Part model, mm, in its own coordinate system. A direction names the side the tool comes from. Give positions to 0.01 mm unless a question says otherwise; leave off trailing zeros. Use a Markdown table: item, result.
Autodesk Inventor part; units mm, degrees
ref_plane "Work Plane1" through (6.245, 5, -17) normal (0, 0, -1) x (-1, 0, 0)
ref_plane "YZ Plane" through (0, 0, 0) normal (1, 0, 0) x (0, 1, 0)
ref_plane "XY Plane" through (0, 0, 0) normal (0, 0, 1) x (1, 0, 0)
sketch "Sketch1" plane through (0, 0, 0) normal (0, 0, 1) x (1, 0, 0)
  point P0 (0, 0)
sketch "Sketch2" plane through (0, 0, 0) normal (1, 0, 0) x (0, 1, 0)
  line L0 (-13.0429, 0) -> (13.0429, 0)
  line L1 (13.0429, 0) -> (13.0429, 3.3095)
  line L2 (13.0429, 3.3095) -> (-13.0429, 3.3095)
  line L3 (-13.0429, 3.3095) -> (-13.0429, 0)
  line L4 (0, 0) -> (0, -15)
  line L5 (0, -15) -> (-8, -15)
  line L6 (-14.2875, 0) -> (14.2875, 0)
  line L7 (14.2875, 0) -> (14.2875, 6.8547)
  line L8 (14.2875, 6.8547) -> (-14.2875, 6.8547)
  line L9 (-14.2875, 6.8547) -> (-14.2875, 0)
  spline S0 degree 4 poles (-14.2875, 0) (-14.2875, -4.9566) (-13.3423, -10.7623) (-11.8115, -15) (-8, -15) knots 0 0 0 0 0 1 1 1 1 1
  point P0 (-12.3627, -11.4481)
  dimension "d1" = 26.0858
  dimension "d2" = 8
  dimension "d3" = 15
  dimension "d4" = 28.575
revolve "Revolution1" add sketch "Sketch2" angle 360 about axis through (0, 0, 0) along (0, 0, -1) contours L0 L4 L5 S0 L6
sketch "Sketch3" plane through (0, 0, 0) normal (0, 0, 1) x (1, 0, 0)
  circle A0 centre (0, 0) radius 14.2875
  circle A1 centre (0, 0) radius 13.0429
  circle A2 centre (0, 0) radius 11
  point P0 (0, -14.2875)
  dimension "d6" = 26.0858
  dimension "d7" = 22
extrude "Extrusion1" add sketch "Sketch3" along normal blind 5 contours A1
hole "Hole1" at (0, 0, 0) direction (0, 0, -1) diameter 3 end through all
sketch "Sketch6" plane through (0, 0, 0) normal (0, 0, 1) x (1, 0, 0)
  circle A0 centre (0, 0) radius 12
  point P0 (4.074, -8.737)
  point P1 (4.82, 8.349)
  point P2 (-9.494, -1.674)
  dimension "d22" = -8.737
  dimension "d23" = 8.349
  dimension "d24" = 1.674
  dimension "d25" = 4.074
  dimension "d26" = 4.82
hole "Hole2" at (-9.494, -1.674, 0) at (4.82, 8.349, 0) at (4.074, -8.737, 0) direction (0, 0, -1) diameter 1.7 end through all
sketch "Sketch8" plane through (0, 0, 0) normal (0, 1, 0) x (-1, 0, 0)
  point P0 (0, 0)
sketch "Sketch9" plane through (0, 0, -15) normal (0, 0, -1) x (-1, 0, 0)
  circle A0 centre (0, 0) radius 1.5
  line L0 (-10.3562, 5) -> (-3, 5)
  line L1 (-3, 5) -> (-3, -5)
  line L2 (-3, -5) -> (-10.3562, -5)
  line L3 (20.0025, 0) -> (-20.0025, 0)
  line L4 (0, -20.0025) -> (0, 20.0025)
  circle A1 centre (-4.82, 8.349) radius 0.85
  circle A2 centre (-4.074, -8.737) radius 0.85
  circle A3 centre (0, 0) radius 8
  arc A4 (-10.3562, 5) -> (-10.3562, -5) centre (0, 0) ccw
  point P0 (0, -8)
  point P1 (-10.7619, 0)
  dimension "d34" = 3
  dimension "d35" = 8.349
  dimension "d36" = 8.737
  dimension "d37" = 10
extrude "Extrusion2" cut sketch "Sketch9" against normal through all contours L3 A3 L0 L1 | L1 L2 A3 L3 | A3 L3 A4 L0 | L2 A4 L3 A3
sketch "Sketch10" plane through (6.245, 5, -15) normal (0, 0, -1) x (-1, 0, 0)
  arc A0 (2.1327, 3.8197) -> (2.1327, 3.8197) centre (2.1327, 3.8197) ccw
  arc A1 (3.0175, -13.6604) -> (3.0175, -13.6604) centre (3.0175, -13.6604) ccw
  arc A2 (16.4746, -6.2481) -> (16.4746, -6.2481) centre (16.4746, -6.2481) ccw
  circle A3 centre (1.425, 3.349) radius 0.85
  circle A4 centre (2.171, -13.737) radius 2.5
  circle A5 centre (2.171, -13.737) radius 0.85
  circle A6 centre (15.739, -6.674) radius 2.5
  circle A7 centre (15.739, -6.674) radius 0.85
  circle A8 centre (1.425, 3.349) radius 2.5
  dimension "d43" = 5
  dimension "d44" = 5
  dimension "d59" = 5
ref_plane "Work Plane1" through (6.245, 5, -17) normal (0, 0, -1) x (-1, 0, 0)
sketch "Sketch11" plane through (6.245, 5, -17) normal (0, 0, -1) x (-1, 0, 0)
  arc A0 (2.1327, 3.8197) -> (2.1327, 3.8197) centre (2.1327, 3.8197) ccw
  arc A1 (16.4746, -6.2481) -> (16.4746, -6.2481) centre (16.4746, -6.2481) ccw
  arc A2 (3.0175, -13.6604) -> (3.0175, -13.6604) centre (3.0175, -13.6604) ccw
  circle A3 centre (1.425, 3.349) radius 2.5
  circle A4 centre (1.425, 3.349) radius 0.85
  circle A5 centre (2.171, -13.737) radius 2.5
  circle A6 centre (15.739, -6.674) radius 2.5
  circle A7 centre (15.739, -6.674) radius 0.85
  circle A8 centre (2.171, -13.737) radius 0.85
  point P0 (6.245, -5)
  dimension "d61" = 5
  dimension "d62" = 5
  dimension "d63" = 5
hole "Hole5" at (4.82, 8.349, -17) at (-9.494, -1.674, -17) at (4.074, -8.737, -17) direction (0, 0, 1) diameter 5 depth 10
sketch "Sketch12" plane through (-9.494, -1.674, -7) normal (0, 0, -1) x (-1, 0, 0)
  circle A0 centre (0, 0) radius 0.85
  circle A1 centre (-14.314, 10.023) radius 0.85
  circle A2 centre (-13.568, -7.063) radius 0.85
  line L0 (-12.264, 8.8394) -> (-14.3141, 7.6559)
  line L1 (-14.3141, 7.6559) -> (-16.364, 8.8395)
  line L2 (-16.364, 8.8395) -> (-16.364, 11.2066)
  line L3 (-16.364, 11.2066) -> (-14.3139, 12.3901)
  line L4 (-14.3139, 12.3901) -> (-12.264, 11.2065)
  line L5 (-12.264, 11.2065) -> (-12.264, 8.8394)
  line L6 (-0.411, -2.3312) -> (-2.2244, -0.8096)
  line L7 (-2.2244, -0.8096) -> (-1.8133, 1.5216)
  line L8 (-1.8133, 1.5216) -> (0.411, 2.3312)
  line L9 (0.411, 2.3312) -> (2.2244, 0.8096)
  line L10 (2.2244, 0.8096) -> (1.8133, -1.5216)
  line L11 (1.8133, -1.5216) -> (-0.411, -2.3312)
  line L12 (-9.494, 1.674) -> (-14.314, 10.023)
  line L13 (-9.494, 1.674) -> (0, 0)
  line L14 (-9.494, 1.674) -> (-13.568, -7.063)
  line L15 (-11.4226, -8.0634) -> (-13.3617, -9.4211)
  line L16 (-13.3617, -9.4211) -> (-15.507, -8.4208)
  line L17 (-15.507, -8.4208) -> (-15.7134, -6.0626)
  line L18 (-15.7134, -6.0626) -> (-13.7743, -4.7049)
  line L19 (-13.7743, -4.7049) -> (-11.629, -5.7052)
  line L20 (-11.629, -5.7052) -> (-11.4226, -8.0634)
  dimension "d71" = 4.1
  dimension "d72" = 4.1
  dimension "d73" = 4.1
extrude "Extrusion3" cut sketch "Sketch12" against normal blind 2 contours L7 L8 L9 L10 L11 L6 | A2 | L19 L20 L15 L16 L17 L18 | L0 L1 L2 L3 L4 L5
ref_plane "Work Plane2" through (0, 13.0429, 0) normal (0, 1, 0) x (-1, 0, 0)
sketch "Sketch13" plane through (0, 13.0429, 0) normal (0, 1, 0) x (-1, 0, 0)
  line L0 (-13.0429, 5) -> (13.0429, 5)
  line L1 (-13.0429, 0) -> (13.0429, 0)
  line L2 (0, -19.0003) -> (0, 9.0001)
  point P0 (0, 0)
  point P1 (0, 2.5)
  dimension "d76" = 2.5
hole "Hole6" at (0, 13.0429, 2.5) direction (0, -1, 0) diameter 1.694 end through all
ref_plane "Work Plane3" through (0, -3.5, 0) normal (0, 1, 0) x (-1, 0, 0)
properties part number "Handle_2_Back"
1. Drill centre lines: L1, parallel to X at y = -3.75, z = -9.5; L2, parallel to X at y = 0, z = -8; L3, parallel to Y at x = -3, z = 2. Where is each one in solid material? Low to high.
Findings below:
| item | result |
|---|---|
| L1 | -12.51 to -10.89, -8.1 to 3, 10.87 to 12.51 |
| L2 | -13.45 to -11.35, -7.64 to -1.5, 1.5 to 3, 11.5 to 13.45 |
| L3 | -12.69 to -10.58, 10.58 to 12.69 |
2. Cut at B-B, the plane x = 0. State how many separate pieces and enclosed holes the cut face has, then the cut area to 3 significant figures.
Findings below:
| item | result |
|---|---|
| separate pieces | 4 |
| enclosed holes | 0 |
| area | 361 mm2 |
3. Tool access for faces 3 (the flat face through (7, -5, -7)), 4 (the flat face through (-9, -7, 5)), 5 (the flat face through (3.223, -6.872, -6.014)): list every direction of +Z, -Z, +X, -X, +Y, -Y with a clear straight run to the whole face (end or side of a thin tool).
Findings below:
| item | result |
|---|---|
| face 3 | +Z, -Z |
| face 4 | +Z, +X, -X, +Y, -Y |
| face 5 | -Z |
4. Two-plate mould, pull along Y, no slides. Class faces 1 (the flat face through (-3, 0, -15)), 2 (the cylindrical face through (11.5, 0.1, -4.1)): released by +Y, released by -Y, zero draft, split by the parting line, or undercut.
Findings below:
| item | result |
|---|---|
| face 1 | zero draft |
| face 2 | undercut |
5. Drop flat-ended pins along their axis: P1, Ø1.3, axis at x = -8.5, y = -1.5, coming from the -Z side; P2, Ø1.5, axis at x = 11, z = -1, coming from the +Y side; P3, Ø8.5, axis at x = 0, y = 1, coming from the +Z side. Give the stop position or say it passes through.
Findings below:
| item | result |
|---|---|
| P1 | z = -5 |
| P2 | y = 9.93 |
| P3 | z = 0 |
